Work out the finished part from the listing and answer in its coordinate system (mm). Face numbers are marked on the shaded views. A direction names the side the tool comes from. Give positions to 0.01 mm unless a question says otherwise; leave off trailing zeros. Loops run counter-clockwise (first coordinate to the right, second up) from the corner with the lowest first, then second, coordinate; pieces in that order, holes last. Notation, with made-up numbers: (-22, -17.75) - (-8, -17.75) arc R29 cw to (-8, 7.25) - close; hole circle Ø8 at (-3.5, 21.25). An arc over 180 degrees is marked (long way). One line per question, with ' | ' between items. Start each with the question number.
1. For a pull along X with two mould halves and no side action, classify the marked faces 3, 4 and 5 as released by +X, released by -X, zero draft, split by the parting line, or undercut.
2. Each of these flat-tipped pins is pushed along its axis until it touches: pin 1 (8 mm diameter, centred on y = -11.5, z = 11.5, fed in from +X); pin 2 (1.9 mm diameter, centred on y = 1, z = 13, fed in from +X); pin 3 (5 mm diameter, centred on x = 19, z = 6.5, fed in from -Y); pin 4 (1.9 mm diameter, centred on x = 0, y = -0.5, fed in from +Z). Where does it stop, or does it pass through?
3. Section B-B (z = 9) is taken. Determine the outline of the cut face in (x, y).
4. Section D-D (z = 1) is taken. Determine the outline of the cut face in (x, y).
5. Section C-C (y = -9.5) is taken. Give the number of separate pieces and of enclosed holes in the cut face, plus the area to 3 significant figures.
6. Which of the six approach directions +Z, -Z, +X, -X, +Y, -Y give full straight-line access (tool end or side, diameter ignored) to the marked faces 1 and 2?
7. Section A-A (x = 0) is taken. Determine the outline of the cut face in (y, z), plus the area to 3 significant figures.
8. Find the intervals of material crossed by line 1 (X direction, y = 12, z = 14.25); line 2 (X direction, y = -12, z = 9.5); line 3 (X direction, y = 0.5, z = 1), in increasing order.
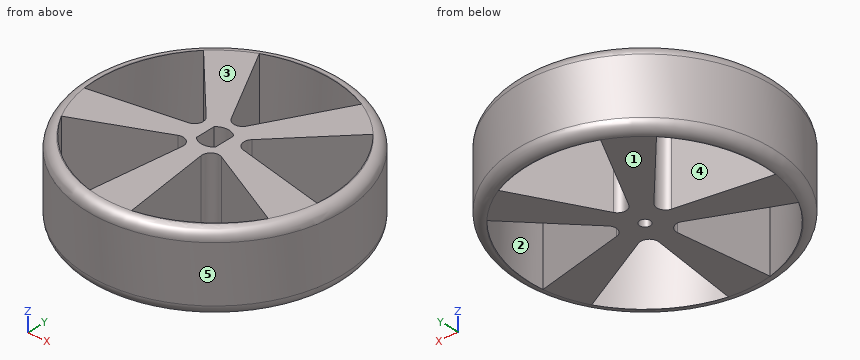
from build123d import *

# Parameters (mm, degrees)
SKETCH1_R           = 25
BOSS_EXTRUDE1_DEPTH = 15
FILLET1_R           = 2
CUT_EXTRUDE1_DEPTH  = 4
SKETCH7_R           = 1.04
CUT_EXTRUDE2_DEPTH  = 39.405728804
CUT_EXTRUDE3_REACH  = 40.406
CIRPATTERN1_COUNT   = 5


with BuildPart() as part:
    # Sketch1 → Boss-Extrude1 (new body)
    with BuildSketch(Plane.XY):
        Circle(SKETCH1_R)
    extrude(amount=BOSS_EXTRUDE1_DEPTH)

    # Fillet1
    fillet1_edges = [part.edges().sort_by_distance(p)[0] for p in [
        (-25, 0, 0),
        (-25, 0, 15),
    ]]
    fillet(fillet1_edges, radius=FILLET1_R)

    # Sketch4 → Cut-Extrude1 (cut)
    with BuildSketch(Plane.XY.offset(15)):
        with BuildLine():
            Line((-1.902969848, 1.941233493), (-1.902969848, -1.941233493))
            ThreePointArc((-1.902969848, -1.941233493), (-0.030378036, -2.71822716), (1.859110772, -1.983277302))
            Line((1.859110772, -1.983277302), (1.859110772, 1.983277302))
            ThreePointArc((1.859110772, 1.983277302), (-0.030378036, 2.71822716), (-1.902969848, 1.941233493))
        make_face()
    extrude(amount=-CUT_EXTRUDE1_DEPTH, mode=Mode.SUBTRACT)

    # Sketch7 → Cut-Extrude2 (cut, through all)
    with BuildSketch(Plane.XY.offset(15)):
        Circle(SKETCH7_R)
    extrude(amount=-CUT_EXTRUDE2_DEPTH, mode=Mode.SUBTRACT)

    # Sketch8 → Cut-Extrude3 (cut, up to next)
    with BuildSketch(Plane(origin=(0, 0, 0), x_dir=(-1, 0, 0), z_dir=(0, 0, -1)), mode=Mode.PRIVATE) as cut_extrude3_sk1:
        with BuildLine():
            Line((-1.5, 5.179174375), (-10, 20.712315177))
            ThreePointArc((-10, 20.712315177), (0, 22.821540356), (10, 20.712315177))
            Line((10, 20.712315177), (1.5, 5.179174375))
            ThreePointArc((1.5, 5.179174375), (0, 4.290100966), (-1.5, 5.179174375))
        make_face()
    cut_extrude3_tool1 = extrude(cut_extrude3_sk1.sketch, amount=-CUT_EXTRUDE3_REACH, mode=Mode.PRIVATE) & part.part
    cut_extrude3 = cut_extrude3_tool1.solids().sort_by_distance((0, 15.677953, 0))[0]
    add(cut_extrude3, mode=Mode.SUBTRACT)

    # CirPattern1: Cut-Extrude3 ×5 about axis
    cirpattern1_axis = Axis((0, 0, 0), (0, 0, 1))
    for i in range(1, CIRPATTERN1_COUNT):
        add(cut_extrude3.rotate(cirpattern1_axis, i * 360 / CIRPATTERN1_COUNT), mode=Mode.SUBTRACT)


solid = part.part
Conclusion:
1) face 3: zero draft | face 4: undercut | face 5: split by the parting line
2) pin 1: x = 23.85 | pin 2: x = 25 | pin 3: y = -18.78 | pin 4: z = 11
3) outline: circle Ø50 at (0, 0); hole (-22.79, -3.11) - (-5.39, 0.17) arc R1.71 ccw to (-4.46, 3.03) - (-16.61, 15.91) arc R24.76 ccw to start; hole (-20.26, -10.88) arc R24.76 ccw to (-4.08, -22.63) - (-1.83, -5.07) arc R1.71 ccw to (-4.26, -3.31) - close; hole (-10, 20.71) - (-1.5, 5.18) arc R1.71 ccw to (1.5, 5.18) - (10, 20.71) arc R24.76 ccw to start; hole circle Ø2.08 at (0, 0); hole (1.83, -5.07) - (4.08, -22.63) arc R24.76 ccw to (20.26, -10.88) - (4.26, -3.31) arc R1.71 ccw to start; hole (4.46, 3.03) arc R1.71 ccw to (5.39, 0.17) - (22.79, -3.11) arc R24.76 ccw to (16.61, 15.91) - close
4) outline: circle Ø49.46 at (0, 0); hole (-22.79, -3.11) - (-5.39, 0.17) arc R1.71 ccw to (-4.46, 3.03) - (-16.61, 15.91) arc R24.76 ccw to start; hole (-20.26, -10.88) arc R24.76 ccw to (-4.08, -22.63) - (-1.83, -5.07) arc R1.71 ccw to (-4.26, -3.31) - close; hole (-10, 20.71) - (-1.5, 5.18) arc R1.71 ccw to (1.5, 5.18) - (10, 20.71) arc R24.76 ccw to start; hole circle Ø2.08 at (0, 0); hole (1.83, -5.07) - (4.08, -22.63) arc R24.76 ccw to (20.26, -10.88) - (4.26, -3.31) arc R1.71 ccw to start; hole (4.46, 3.03) arc R1.71 ccw to (5.39, 0.17) - (22.79, -3.11) arc R24.76 ccw to (16.61, 15.91) - close
5) separate pieces: 3 | enclosed holes: 0 | area: 242 mm²
6) face 1: -Z, +X, -X, +Y, -Y | face 2: +Z, -Z
7) outline: (-25, 2) arc R2 ccw to (-23, 0) - (-1.04, 0) - (-1.04, 11) - (-2.72, 11) - (-2.72, 15) - (-23, 15) arc R2 ccw to (-25, 13) - close; (1.04, 0) - (4.29, 0) - (4.29, 15) - (2.72, 15) - (2.72, 11) - (1.04, 11) - close; (22.82, 0) - (23, 0) arc R2 ccw to (25, 2) - (25, 13) arc R2 ccw to (23, 15) - (22.82, 15) - close | area: 424 mm²
8) line 1: -21.43 to -19.47, -12.92 to -5.23, 5.23 to 12.92, 19.47 to 21.43 | line 2: -21.93 to -19.57, -2.72 to 2.72, 19.57 to 21.93 | line 3: -24.73 to -22.89, -4.66 to -0.91, 0.91 to 4.66, 22.89 to 24.73
